Check sheet for the modelled part. Datum: model origin and axes. Units: mm. A direction names the side the tool comes from. Round coordinates to 2 decimals unless told otherwise and drop trailing zeros. Loops run counter-clockwise (first coordinate to the right, second up) from the corner with the lowest first, then second, coordinate; pieces in that order, holes last. Notation, with made-up numbers: (58, 16.5) -> (79, 16.5) arc R20 cw to (79, 35.5) -> close; hole circle Ø2 at (72.25, -35). An arc over 180 degrees is marked (long way). One line per item, written item: value. Start each with the question number.
1. Go/stop test with flat-tipped pins: pin 1 (4 mm diameter, centred on x = 1, y = -21, fed in from +Z); pin 2 (8 mm diameter, centred on x = -16.5, z = -8, fed in from +Y); pin 3 (1 mm diameter, centred on x = -2, y = -136, fed in from +Z); pin 4 (1 mm diameter, centred on x = -12, y = -66, fed in from +Z). Record where each tip stops, or that it passes through.
2. Cross-section at D-D on y = -28. Record the cut outline in (x, z), then the cut area to 3 significant figures.
3. Cross-section at B-B on x = -7.64. Record the cut outline in (y, z).
4. Set-up check for faces 1 (the face through (-3.5, -92.12, -9.2)), 2 (the face through (-8, 0, 0)): record each of +Z, -Z, +X, -X, +Y, -Y from which the full face is reachable in a straight line by a thin tool's end or side.
5. Material ranges on L1, parallel to Y at x = -16.75, z = 3; L2, parallel to Y at x = -14.75, z = -9.75; L3, parallel to Z at x = -12.5, y = -55.5, recorded low to high.
6. Cross-section at C-C on y = -114. Record the cut outline in (x, z), then the cut area to 3 significant figures.
7. Cross-section at A-A on z = 0. Record the cut outline in (x, y), then the cut area to 3 significant figures.
from build123d import *

# Parameters (mm, degrees)
F0_R     = 12.319
F1_DEPTH = 46.219999
F2_R     = 11.303
F3_DEPTH = 45.90001
F4_R     = 9.906
F5_DEPTH = 34.879999
F6_R     = 8.509
F7_DEPTH = 18.299999
F8_R     = 7.366
F9_DEPTH = 18.28


with BuildPart() as f1:
    # F0 (on Front) → F1 (new body)
    with BuildSketch(Plane.XZ):
        with Locations((-7.64, 0)):
            Circle(F0_R)
    extrude(amount=F1_DEPTH)

    # F2 (on face) → F3 (join)
    with BuildSketch(Plane.XZ.offset(46.219999)):
        with Locations((-7.64, 0)):
            Circle(F2_R)
    extrude(amount=F3_DEPTH)

    # F4 (on face) → F5 (join)
    with BuildSketch(Plane.XZ.offset(92.120009)):
        with Locations((-7.64, 0)):
            Circle(F4_R)
    extrude(amount=F5_DEPTH)

    # F6 (on face) → F7 (join)
    with BuildSketch(Plane.XZ.offset(127.000008)):
        with Locations((-7.64, 0)):
            Circle(F6_R)
    extrude(amount=F7_DEPTH)

    # F8 (on face) → F9 (join)
    with BuildSketch(Plane.XZ.offset(145.300007)):
        with Locations((-7.64, 0)):
            Circle(F8_R)
    extrude(amount=F9_DEPTH)


solid = f1.part
Taken from the geometry:
1. pin 1: stops at z = 10.38
1. pin 2: stops at y = 0
1. pin 3: stops at z = 6.78
1. pin 4: stops at z = 10.62
2. outline: circle Ø24.64 at (-7.64, 0)
2. area: 477 mm2
3. outline: (-163.58, -7.37) -> (-145.3, -7.37) -> (-145.3, -8.51) -> (-127, -8.51) -> (-127, -9.91) -> (-92.12, -9.91) -> (-92.12, -11.3) -> (-46.22, -11.3) -> (-46.22, -12.32) -> (0, -12.32) -> (0, 12.32) -> (-46.22, 12.32) -> (-46.22, 11.3) -> (-92.12, 11.3) -> (-92.12, 9.91) -> (-127, 9.91) -> (-127, 8.51) -> (-145.3, 8.51) -> (-145.3, 7.37) -> (-163.58, 7.37) -> close
4. face 1: -Y
4. face 2: +Z, -Z, +X, -X, +Y
5. L1: y = -127 to 0
5. L2: y = -46.22 to 0
5. L3: z = -10.2 to 10.2
6. outline: circle Ø19.81 at (-7.64, 0)
6. area: 308 mm2
7. outline: (-19.96, -46.22) -> (-18.94, -46.22) -> (-18.94, -92.12) -> (-17.55, -92.12) -> (-17.55, -127) -> (-16.15, -127) -> (-16.15, -145.3) -> (-15.01, -145.3) -> (-15.01, -163.58) -> (-0.27, -163.58) -> (-0.27, -145.3) -> (0.87, -145.3) -> (0.87, -127) -> (2.27, -127) -> (2.27, -92.12) -> (3.66, -92.12) -> (3.66, -46.22) -> (4.68, -46.22) -> (4.68, 0) -> (-19.96, 0) -> close
7. area: 3,450 mm2
